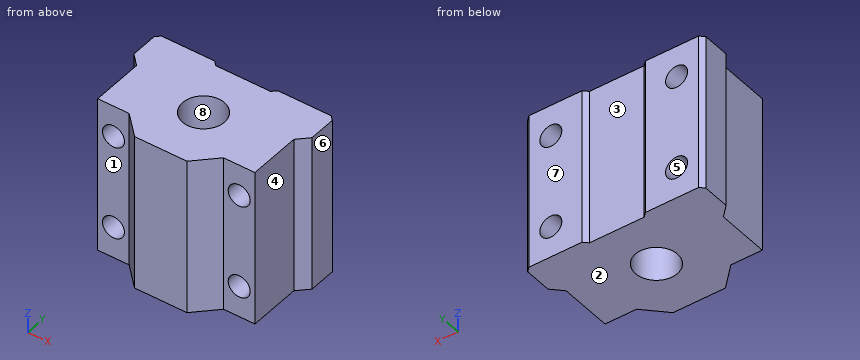
```python
from build123d import *

# Parameters (mm, degrees)
SKETCH_1_R          = 4
EXTRUDE_1_DEPTH     = 30
SKETCH_2_R          = 2.1
CUT_EXTRUDE_1_DEPTH = 30


with BuildPart() as part:
    # 草图1 → 凸台-拉伸1 (new body)
    with BuildSketch(Plane.XY):
        Polygon((5, -11), (-5, -11), (-9, -7), (-15, -7), (-15, 3), (-17, 5), (-17, 10.2), (-16.2, 11), (-6.034999107, 11), (-5.234999107, 10.2), (5.234999107, 10.2), (6.034999107, 11), (16.2, 11), (17, 10.2), (17, 5), (15, 3), (15, -7), (9, -7), align=None)
        Circle(SKETCH_1_R, mode=Mode.SUBTRACT)
    extrude(amount=EXTRUDE_1_DEPTH)

    # 草图2 → 切除-拉伸1 (cut)
    with BuildSketch(Plane(origin=(0, 11, 0), x_dir=(1, 0, 0), z_dir=(0, 1, 0))):
        with Locations(Location((-12, -6, 0), (0, 0, 270))):
            Circle(SKETCH_2_R)
        with Locations(Location((-12, -24, 0), (0, 0, 270))):
            Circle(SKETCH_2_R)
        with Locations(Location((12, -6, 0), (0, 0, 180))):
            Circle(SKETCH_2_R)
        with Locations(Location((12, -24, 0), (0, 0, 180))):
            Circle(SKETCH_2_R)
    extrude(amount=-CUT_EXTRUDE_1_DEPTH, mode=Mode.SUBTRACT)


solid = part.part
```
Read the model definition and answer for the solid it produces. Units are mm, in the model's axes. Face numbers are marked on the shaded views. A direction names the side the tool comes from. Give positions to 0.01 mm unless a question says otherwise; leave off trailing zeros. Loops run counter-clockwise (first coordinate to the right, second up) from the corner with the lowest first, then second, coordinate; pieces in that order, holes last.
Item 1: The part is cut by section D-D (x = 12). Write down the section's boundary in (y, z), and give its area (3 significant figures).
Item 2: Find the intervals of material crossed by line 1 along Z through (x, y) = (12, 1.25); line 2 along Y through (x, z) = (0, 18); line 3 along X through (y, z) = (-0.25, 11.5), in increasing order.
Item 3: Each of these flat-tipped pins is pushed along its axis until it touches: pin 1 Ø8.5 at (x, z) = (-1.5, 15.5) entering from +Y (3 decimals); pin 2 Ø3 at (y, z) = (-0.5, 12) entering from +X; pin 3 Ø4 at (x, z) = (-12, 24) entering from +Y; pin 4 Ø2 at (x, z) = (0.5, 24.5) entering from +Y. Where does it stop, or does it pass through?
Item 4: The mould has two halves that part along X. Classify the marked faces 5, 6, 7 and 8: released by +X, released by -X, zero draft, split by the parting line, or undercut.
Item 5: The part is cut by section C-C (x = 0). Write down the section's boundary in (y, z), and give its area (3 significant figures).
Item 6: The part is cut by section A-A (z = 6). Write down the section's boundary in (x, y) (3 decimals).
Item 7: For the marked faces 1, 2, 3 and 4, determine the directions among +Z, -Z, +X, -X, +Y, -Y from which every point of the face is accessible in a straight line to the end or side of a thin tool.
Item 8: The part is cut by section B-B (y = 7.5). Write down the section's boundary in (x, z).
Taken from the geometry:
1. outline: (-7, 0) - (11, 0) - (11, 3.9) - (-7, 3.9) - close; (-7, 8.1) - (11, 8.1) - (11, 21.9) - (-7, 21.9) - close; (-7, 26.1) - (11, 26.1) - (11, 30) - (-7, 30) - close
1. area: 389 mm2
2. line 1: z = 0 to 3.9, 8.1 to 21.9, 26.1 to 30
2. line 2: y = -11 to -4, 4 to 10.2
2. line 3: x = -15 to -3.99, 3.99 to 15
3. pin 1: stops at y = 10.715
3. pin 2: stops at x = 15
3. pin 3: passes through
3. pin 4: stops at y = 10.2
4. face 5: undercut
4. face 6: released by +X
4. face 7: zero draft
4. face 8: undercut
5. outline: (-11, 0) - (-4, 0) - (-4, 30) - (-11, 30) - close; (4, 0) - (10.2, 0) - (10.2, 30) - (4, 30) - close
5. area: 396 mm2
6. outline: (-17, 5) - (-15, 3) - (-15, -7) - (-14.1, -7) - (-14.1, 11) - (-16.2, 11) - (-17, 10.2) - close; (-9.9, -7) - (-9, -7) - (-5, -11) - (5, -11) - (9, -7) - (9.9, -7) - (9.9, 11) - (6.035, 11) - (5.235, 10.2) - (-5.235, 10.2) - (-6.035, 11) - (-9.9, 11) - close; (14.1, -7) - (15, -7) - (15, 3) - (17, 5) - (17, 10.2) - (16.2, 11) - (14.1, 11) - close; hole circle Ø8 at (0, 0)
7. face 1: +Z, -Z, -X, -Y
7. face 2: -Z, +X, -X, +Y, -Y
7. face 3: +Z, -Z, +Y
7. face 4: +Z, -Z, +X, -Y
8. outline: (-17, 0) - (17, 0) - (17, 30) - (-17, 30) - close; hole circle Ø4.2 at (-12, 6); hole circle Ø4.2 at (-12, 24); hole circle Ø4.2 at (12, 6); hole circle Ø4.2 at (12, 24)
